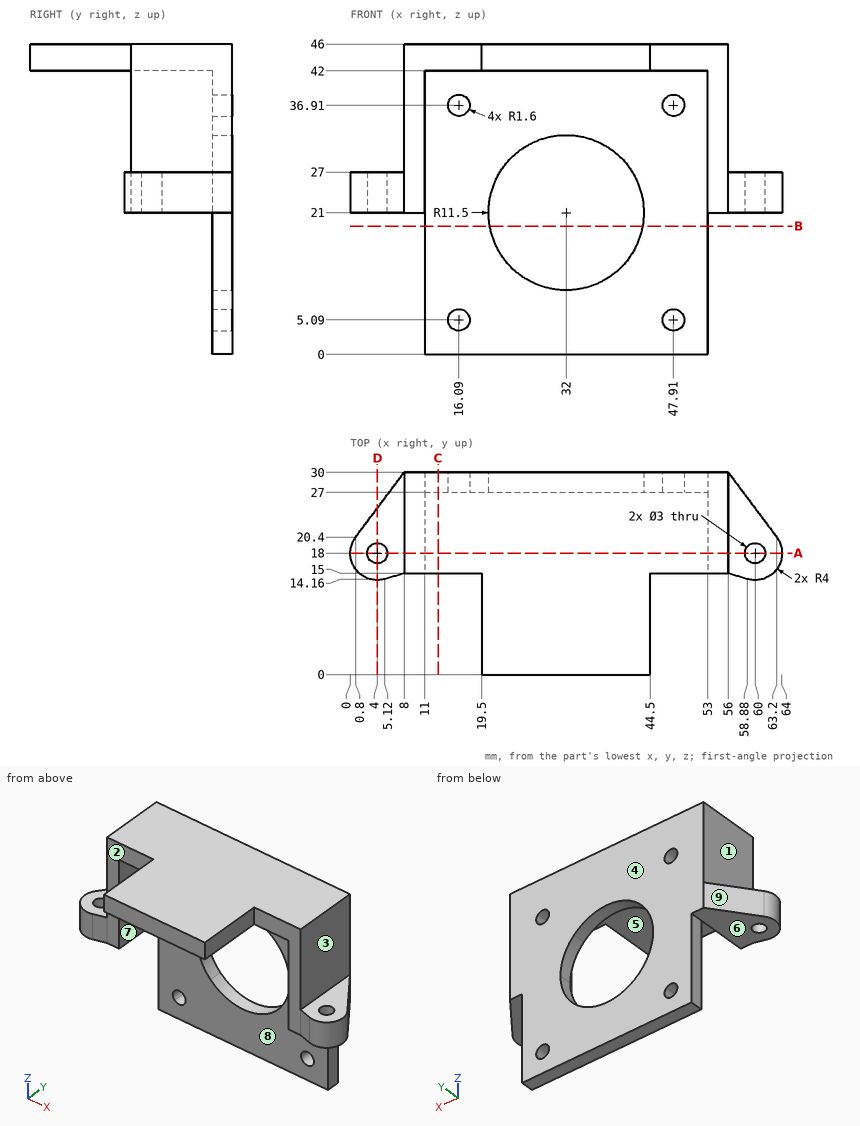
Geometry check sheet. Reference: drawing and pictorial views, mm from the part's lowest x, y, z. A direction names the side the tool comes from. Round coordinates to 2 decimals unless told otherwise and drop trailing zeros. Loops run counter-clockwise (first coordinate to the right, second up) from the corner with the lowest first, then second, coordinate; pieces in that order, holes last. Notation, with made-up numbers: (23, -11) -> (54, -11) arc R19 ccw to (54, 25) -> close; hole circle Ø2 at (23, -19). An arc over 180 degrees is marked (long way). Answer as a JSON object with one key per item and string values. Group by question number.
Item 1: Cross-section at A-A, the plane y = 18. Record the cut outline in (x, z).
Item 2: Cross-section at C-C, the plane x = 13. Record the cut outline in (y, z), plus the area to 3 significant figures.
Item 3: Depth check by flat-ended pin: pin 1 Ø3.5 at (x, z) = (49, 30.5) entering from -Y; pin 2 Ø3 at (y, z) = (11, 43.5) entering from -X; pin 3 Ø2.5 at (y, z) = (28.5, 10.5) entering from +X. Enter the tip coordinate at first touch or a pass-through.
Item 4: Cross-section at D-D, the plane x = 4. Record the cut outline in (y, z).
Item 5: Release check for a two-part mould opening along X. For the marked faces 6, 7, 8 and 9 record: pulls with the +X half, pulls with the -X half, needs draft (parallel to the pull), parting line crosses it, or undercut.
Item 6: Thickness scan on line 1 along X through (y, z) = (18, 24.1); line 2 along X through (y, z) = (20.75, 40); line 3 along Y through (x, z) = (29.5, 35). Record the ranges inside material, lowest first.
Item 7: Cross-section at B-B, the plane z = 19. Record the cut outline in (x, y).
Item 8: Set-up check for the marked faces 1, 2, 3, 4 and 5: record each of +Z, -Z, +X, -X, +Y, -Y from which the full face is reachable in a straight line by a thin tool's end or side.
Determined:
{
 "1": {"outline": "(0, 21) -> (2.5, 21) -> (2.5, 27) -> (0, 27) -> close; (5.5, 21) -> (11, 21) -> (11, 42) -> (53, 42) -> (53, 21) -> (58.5, 21) -> (58.5, 27) -> (56, 27) -> (56, 46) -> (8, 46) -> (8, 27) -> (5.5, 27) -> close; (61.5, 21) -> (64, 21) -> (64, 27) -> (61.5, 27) -> close"},
 "2": {"outline": "(15, 42) -> (27, 42) -> (27, 0) -> (30, 0) -> (30, 46) -> (15, 46) -> close", "area": "186 mm²"},
 "3": {"pin 1": "stops at y = 27", "pin 2": "stops at x = 19.5", "pin 3": "stops at x = 53"},
 "4": {"outline": "(14, 21) -> (16.5, 21) -> (16.5, 27) -> (14, 27) -> close; (19.5, 21) -> (24.67, 21) -> (24.67, 27) -> (19.5, 27) -> close"},
 "5": {"face 6": "needs draft", "face 7": "undercut", "face 8": "undercut", "face 9": "pulls with the -X half"},
 "6": {"line 1": "x = 0 to 2.5, 5.5 to 11, 53 to 58.5, 61.5 to 64", "line 2": "x = 8 to 11, 53 to 56", "line 3": "y = 27 to 30"},
 "7": {"outline": "(11, 27) -> (20.68, 27) -> (20.68, 30) -> (11, 30) -> close; (43.32, 27) -> (53, 27) -> (53, 30) -> (43.32, 30) -> close"},
 "8": {"face 1": "+Z, -X, +Y, -Y", "face 2": "+Z, -Z, -Y", "face 3": "+Z, +X, +Y, -Y", "face 4": "+Z, -Z, +X, -X, +Y", "face 5": "-Z, -Y"}
}
